Verification items for this drawing (mm, ordinates from the low corner). A direction names the side the tool comes from. Round coordinates to 2 decimals unless told otherwise and drop trailing zeros. Order: outer loops, then holes, each group sorted by start corner. A loop starts at its lowest first (then second) coordinate and runs counter-clockwise, first axis right, second up. Notation, with made-up numbers: M -8,39 L 46,39 A8 cw 46,48 Z; hole C 24.5,76.5 d2. An arc over 180 degrees is marked long. One line per item, written item: value. Start each with the question number.
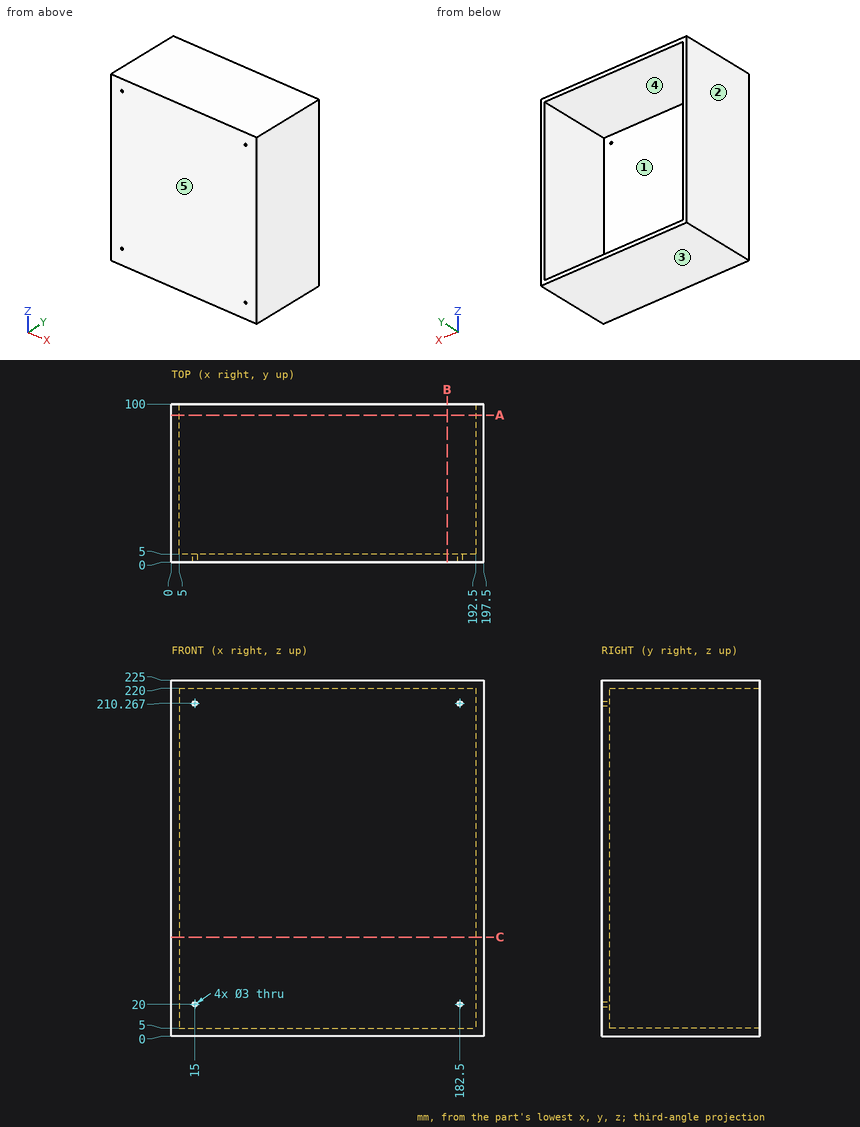
1. Tool access check on the marked faces 4 and 5. Record the directions out of +Z, -Z, +X, -X, +Y, -Y that give a thin tool (end or side, any length) a straight path to the whole face; none if there is none.
2. Scan lines: line 1 along X through (y, z) = (1.85, 20); line 2 along Z through (x, y) = (15, 3.2); line 3 along X through (y, z) = (80, 33). Record each from-to range of solid material in increasing order.
3. Draft check along Z on the marked faces 1, 2 and 3. Enter one of: released by +Z, released by -Z, zero draft, split by the parting line, or undercut.
4. Depth check by flat-ended pin: pin 1 (3.5 mm diameter, centred on x = 15, z = 210.267, fed in from +Y). Enter the tip coordinate at first touch or a pass-through.
5. Section check C-C (z = 62.5). Record the cut outline in (x, y), and give its area (3 significant figures).
6. Section check B-B (x = 174.5). Record the cut outline in (y, z).
7. Section check A-A (y = 93). Record the cut outline in (x, z), and give its area (4 significant figures).
Geometry check:
1. face 4: +Y
1. face 5: +Z, -Z, +X, -X, -Y
2. line 1: x = 0 to 13.5, 16.5 to 181, 184 to 197.5
2. line 2: z = 0 to 18.5, 21.5 to 208.77, 211.77 to 225
2. line 3: x = 0 to 5, 192.5 to 197.5
3. face 1: undercut
3. face 2: zero draft
3. face 3: released by -Z
4. pin 1: stops at y = 5
5. outline: M 0,0 L 197.5,0 L 197.5,100 L 192.5,100 L 192.5,5 L 5,5 L 5,100 L 0,100 Z
5. area: 1,940 mm²
6. outline: M 0,0 L 100,0 L 100,5 L 5,5 L 5,220 L 100,220 L 100,225 L 0,225 Z
7. outline: M 0,0 L 197.5,0 L 197.5,225 L 0,225 Z; hole M 5,5 L 192.5,5 L 192.5,220 L 5,220 Z
7. area: 4,125 mm²
